Input: part model. Units: mm. Frame: model coordinates. Face numbers are marked on the shaded views. A direction names the side the tool comes from. Round coordinates to 2 decimals unless told otherwise and drop trailing zeros. Loops run counter-clockwise (first coordinate to the right, second up) from the corner with the lowest first, then second, coordinate; pieces in that order, holes last. Notation, with made-up numbers: (79.5, 69) - (84.5, 69) arc R11 cw to (84.5, 78) - close; hole circle Ø4 at (29, 50.25). An arc over 180 degrees is marked (long way). One line per question, with ' | ' between items. Start each with the question number.
Item 1: Section A-A, the plane y = 523. Return loops of the section in (x, z), plus the area to 3 significant figures.
Item 2: Section D-D, the plane y = 545.5. Return loops of the section in (x, z).
Item 3: First-contact query: pin 1 (12 mm diameter, centred on x = -19.5, z = -175.5, fed in from -Y); pin 2 (4 mm diameter, centred on x = -23, z = -218.5, fed in from -Y); pin 3 (5 mm diameter, centred on x = 8, y = 563.5, fed in from -Z); pin 4 (2 mm diameter, centred on x = 12, z = -227, fed in from -Y). Flat tips, straight axial feed; report the tip coordinate or a pass-through.
Item 4: Section B-B, the plane z = -169. Return loops of the section in (x, y), plus the area to 3 significant figures.
Item 5: Section C-C, the plane x = 26. Return loops of the section in (y, z), plus the area to 3 significant figures.
Item 6: Draft query along Y for the marked faces 1, 2, 3 and 4. Return one class per face: pulls with the +Y half, pulls with the -Y half, needs draft (parallel to the pull), parting line crosses it, or undercut.
Item 7: Set-up query: the marked faces 5 and 6. Return all of +Z, -Z, +X, -X, +Y, -Y with unobstructed straight access to the full face (end or side cutting, diameter ignored); none if empty.
Item 8: Material intervals for line 1 along X through (y, z) = (557.5, -209.5); line 2 along Y through (x, z) = (15, -228.5); line 3 along Y through (x, z) = (24, -185), sorted ascending.
```python
from build123d import *

# Parameters (mm, degrees)
BOSS_EXTRUDE1_DEPTH      = 20.832572
BOSS_EXTRUDE1_DEPTH_BACK = 20.832572
SKETCH1_W                = 103.439976
SKETCH1_H                = 10.722102
SKETCH2_R                = 19.704892681
BOSS_EXTRUDE2_DEPTH      = 8.586216


with BuildPart() as part:
    # Sketch1 → Boss-Extrude1 (new, two sides: drawn at the far end of the back side and taken through both)
    with BuildSketch(Plane(origin=(0, 0, 0), x_dir=(0, 0, -1), z_dir=(1, 0, 0)).offset(-BOSS_EXTRUDE1_DEPTH_BACK)):
        with Locations((185.773568, 570.773433)):
            Rectangle(SKETCH1_W, SKETCH1_H)
    extrude(amount=BOSS_EXTRUDE1_DEPTH + BOSS_EXTRUDE1_DEPTH_BACK)

    # Sketch2 → Boss-Extrude2 (add)
    with BuildSketch(Plane(origin=(20.832572, 0, 0), x_dir=(0, 0, -1), z_dir=(1, 0, 0))):
        with BuildLine():
            Line((134.05358, 565.412382), (134.05358, 576.134484))
            Line((134.05358, 576.134484), (237.493556, 576.134484))
            Line((237.493556, 576.134484), (237.493556, 565.412382))
            ThreePointArc((237.493556, 565.412382), (185.773568, 513.692394), (134.05358, 565.412382))
        make_face()
        with Locations((185.811668, 541.18891)):
            Circle(SKETCH2_R, mode=Mode.SUBTRACT)
    boss_extrude2 = extrude(amount=BOSS_EXTRUDE2_DEPTH)

    # Mirror1: Boss-Extrude2 across plane
    add(boss_extrude2.mirror(Plane(origin=(0, 0, 0), x_dir=(0, 0, 1), z_dir=(1, 0, 0))))


solid = part.part
```
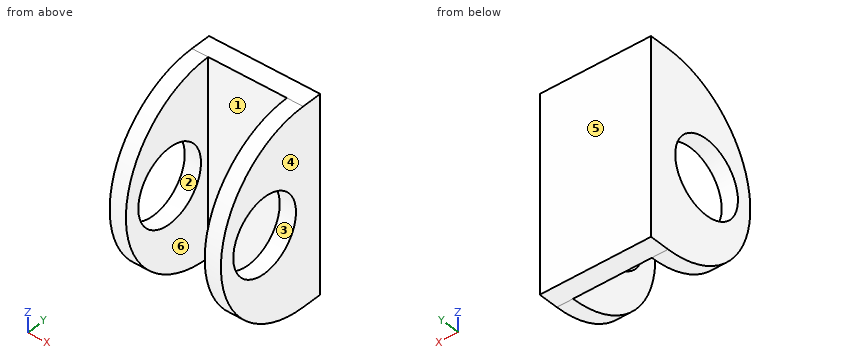
Return value:
1) outline: (-29.42, -215.37) - (-20.83, -215.37) - (-20.83, -193.39) - (-29.42, -193.39) - close; (-29.42, -178.23) - (-20.83, -178.23) - (-20.83, -156.17) - (-29.42, -156.17) - close; (20.83, -215.37) - (29.42, -215.37) - (29.42, -193.39) - (20.83, -193.39) - close; (20.83, -178.23) - (29.42, -178.23) - (29.42, -156.17) - (20.83, -156.17) - close | area: 756 mm2
2) outline: (-29.42, -233.51) - (-20.83, -233.51) - (-20.83, -205.04) - (-29.42, -205.04) - close; (-29.42, -166.58) - (-20.83, -166.58) - (-20.83, -138.04) - (-29.42, -138.04) - close; (20.83, -233.51) - (29.42, -233.51) - (29.42, -205.04) - (20.83, -205.04) - close; (20.83, -166.58) - (29.42, -166.58) - (29.42, -138.04) - (20.83, -138.04) - close
3) pin 1: y = 513.88 | pin 2: y = 523.81 | pin 3: z = -237.49 | pin 4: y = 565.41
4) outline: (-29.42, 516.49) - (-20.83, 516.49) - (-20.83, 530.91) - (-29.42, 530.91) - close; (-29.42, 551.47) - (-20.83, 551.47) - (-20.83, 565.41) - (20.83, 565.41) - (20.83, 551.47) - (29.42, 551.47) - (29.42, 576.13) - (-29.42, 576.13) - close; (20.83, 516.49) - (29.42, 516.49) - (29.42, 530.91) - (20.83, 530.91) - close | area: 1,120 mm2
5) outline: (565.41, -237.49) - (576.13, -237.49) - (576.13, -134.05) - (565.41, -134.05) arc R51.72 ccw to start; hole circle Ø39.41 at (541.19, -185.81) | area: 4,090 mm2
6) face 1: pulls with the -Y half | face 2: undercut | face 3: undercut | face 4: needs draft
7) face 5: +Z, -Z, +X, -X, +Y | face 6: +Z, -Z, -Y
8) line 1: -29.42 to -20.83, 20.83 to 29.42 | line 2: 565.41 to 576.13 | line 3: 513.7 to 521.5, 560.88 to 576.13
